Could you check a few things on this drawing? It's one solid part, dimensions in mm from its lowest x, y, z. A direction names the side the tool comes from. Give positions to 0.01 mm unless a question says otherwise; leave off trailing zeros.
Item 1: I'm going to push flat-ended pins straight in: pin 1 Ø1 at (x, y) = (54, 5) entering from +Z (1 decimal); pin 2 Ø4 at (x, y) = (12.5, 11) entering from +Z (1 decimal); pin 3 Ø1 at (x, y) = (46, 2) entering from -Z. Where does each tip first touch, or does it pass through?
Item 2: Which directions (+Z, -Z, +X, -X, +Y, -Y) give clear straight access to the entire face, cutting with the end or side of a thin tool? Please do the marked faces 1 and 2.
Item 3: If I drill on line 1 along X through (y, z) = (7.5, 1.75); line 2 along Z through (x, y) = (27.5, 3.5) (1 decimal); line 3 along Z through (x, y) = (55.5, 1) (1 decimal), over which ranges is the centre line in solid material (lowest first)?
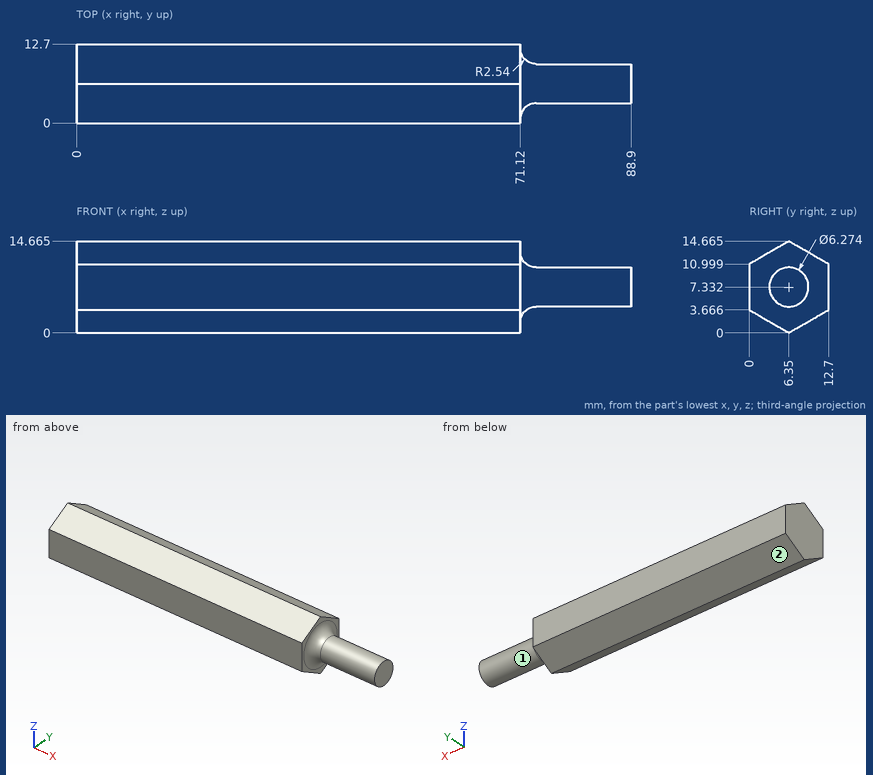
Results list:
1. pin 1: stops at z = 14.2
1. pin 2: stops at z = 13.1
1. pin 3: stops at z = 2.22
2. face 1: +X
2. face 2: -Z, +X, -X, +Y
3. line 1: x = 0 to 71.12
3. line 2: z = 1.6 to 13
3. line 3: z = 3.1 to 11.6
